Verification items for the finished model (mm, model axes). A direction names the side the tool comes from. Coordinates: 2 decimals unless noted, no trailing zeros. Loops run counter-clockwise (first coordinate to the right, second up) from the corner with the lowest first, then second, coordinate; pieces in that order, holes last.
Q1. Go/stop test with flat-tipped pins: P1, Ø3, axis at x = 57, y = 18.5, coming from the +Z side; P2, Ø5, axis at x = 78, z = -46.5, coming from the +Y side; P3, Ø4, axis at y = 19, z = -25, coming from the +X side; P4, Ø3, axis at y = 20.5, z = -59, coming from the +X side. Record where each tip stops, or that it passes through.
Q2. Sectioned sample at B-B (x = 66.5). Enter the section's corners in (y, z), then the cut area to 3 significant figures.
Q3. Sectioned sample at C-C (z = -9). Enter the section's corners in (x, y).
Q4. Sectioned sample at D-D (x = 9). Enter the section's corners in (y, z), then the cut area to 3 significant figures.
Q5. Material ranges on probe 1 along Y at (x, z) = (82, -53); probe 2 along Z at (x, y) = (54, 13.25); probe 3 along Z at (x, y) = (34, 3.5), recorded low to high.
Q6. Mould release check, pull along Z, two halves, no side actions. Record for faces 4 (the face through (60.53, 2.61, -50.89)), 5 (the face through (62.13, 2.85, -43.01)), 6 (the face through (23.49, 2.85, -19.79)): +Z half, -Z half, draft (parallel to the pull), parting line (faces both ways), or undercut.
Q7. Access from +Z, -Z, +X, -X, +Y, -Y to the whole of each face (thin tool, end or side, straight path). Record for faces 1 (the face through (26.5, 13, -20)), 2 (the face through (2.36, 13.73, -20.34)), 3 (the face through (62.13, 23.49, -42.85)).
Q8. Sectioned sample at A-A (y = 13.25). Enter the section's corners in (x, z), then the cut area to 3 significant figures.
```python
from build123d import *

# Parameters (mm, degrees)
BOSS_EXTRUDE1_DEPTH = 26.5
SKETCH3_R           = 10.9
CUT_EXTRUDE1_DEPTH  = 129.322835068
SKETCH4_R           = 10.9
CUT_EXTRUDE2_DEPTH  = 129.322835068
FILLET1_R           = 10


with BuildPart() as part:
    # Sketch2 → Boss-Extrude1 (new body)
    with BuildSketch(Plane(origin=(0, 0, 0), x_dir=(1, 0, 0), z_dir=(0, 1, 0))):
        Polygon((0, 0), (0, 66.5), (106.5, 66.5), (106.5, 40), (26.5, 40), (26.5, 0), align=None)
    extrude(amount=BOSS_EXTRUDE1_DEPTH)

    # Sketch3 → Cut-Extrude1 (cut, through all)
    with BuildSketch(Plane.XY):
        with Locations((13.25, 13.25)):
            Circle(SKETCH3_R)
    extrude(amount=-CUT_EXTRUDE1_DEPTH, mode=Mode.SUBTRACT)

    # Sketch4 → Cut-Extrude2 (cut, through all)
    with BuildSketch(Plane(origin=(106.5, 0, 0), x_dir=(0, 0, -1), z_dir=(1, 0, 0))):
        with Locations((53.25, 13.25)):
            Circle(SKETCH4_R)
    extrude(amount=-CUT_EXTRUDE2_DEPTH, mode=Mode.SUBTRACT)

    # Fillet1
    # the kernel refuses this fillet: 10 mm, written as the material it takes off along each edge
    with BuildSketch(Plane(origin=(106.5, 26.5, -40), x_dir=(0, 0, -1), z_dir=(-1, 0, 0))) as fillet1_piece_1:
        with BuildLine():
            CenterArc((FILLET1_R, FILLET1_R), FILLET1_R, 180, 90)
            Line((0, FILLET1_R), (-FILLET1_R * 0.02, FILLET1_R))
            Line((-FILLET1_R * 0.02, FILLET1_R), (-FILLET1_R * 0.02, -FILLET1_R * 0.02))
            Line((-FILLET1_R * 0.02, -FILLET1_R * 0.02), (FILLET1_R, -FILLET1_R * 0.02))
            Line((FILLET1_R, -FILLET1_R * 0.02), (FILLET1_R, 0))
        make_face()
    extrude(amount=80, mode=Mode.SUBTRACT)
    with BuildSketch(Plane(origin=(0, 26.5, -66.5), x_dir=(0, 0, 1), z_dir=(1, 0, 0))) as fillet1_piece_2:
        with BuildLine():
            CenterArc((FILLET1_R, FILLET1_R), FILLET1_R, 180, 90)
            Line((0, FILLET1_R), (-FILLET1_R * 0.02, FILLET1_R))
            Line((-FILLET1_R * 0.02, FILLET1_R), (-FILLET1_R * 0.02, -FILLET1_R * 0.02))
            Line((-FILLET1_R * 0.02, -FILLET1_R * 0.02), (FILLET1_R, -FILLET1_R * 0.02))
            Line((FILLET1_R, -FILLET1_R * 0.02), (FILLET1_R, 0))
        make_face()
    extrude(amount=106.5, mode=Mode.SUBTRACT)
    with BuildSketch(Plane(origin=(0, 0, -66.5), x_dir=(0, 0, 1), z_dir=(1, 0, 0))) as fillet1_piece_3:
        with BuildLine():
            CenterArc((FILLET1_R, -FILLET1_R), FILLET1_R, 90, 90)
            Line((0, -FILLET1_R), (-FILLET1_R * 0.02, -FILLET1_R))
            Line((-FILLET1_R * 0.02, -FILLET1_R), (-FILLET1_R * 0.02, FILLET1_R * 0.02))
            Line((-FILLET1_R * 0.02, FILLET1_R * 0.02), (FILLET1_R, FILLET1_R * 0.02))
            Line((FILLET1_R, FILLET1_R * 0.02), (FILLET1_R, 0))
        make_face()
    extrude(amount=106.5, mode=Mode.SUBTRACT)
    with BuildSketch(Plane(origin=(106.5, 0, -40), x_dir=(0, 0, -1), z_dir=(-1, 0, 0))) as fillet1_piece_4:
        with BuildLine():
            CenterArc((FILLET1_R, -FILLET1_R), FILLET1_R, 90, 90)
            Line((0, -FILLET1_R), (-FILLET1_R * 0.02, -FILLET1_R))
            Line((-FILLET1_R * 0.02, -FILLET1_R), (-FILLET1_R * 0.02, FILLET1_R * 0.02))
            Line((-FILLET1_R * 0.02, FILLET1_R * 0.02), (FILLET1_R, FILLET1_R * 0.02))
            Line((FILLET1_R, FILLET1_R * 0.02), (FILLET1_R, 0))
        make_face()
    extrude(amount=80, mode=Mode.SUBTRACT)
    with BuildSketch(Plane(origin=(26.5, 0, -40), x_dir=(-1, 0, 0), z_dir=(0, 0, 1))) as fillet1_piece_5:
        with BuildLine():
            CenterArc((FILLET1_R, -FILLET1_R), FILLET1_R, 90, 90)
            Line((0, -FILLET1_R), (-FILLET1_R * 0.02, -FILLET1_R))
            Line((-FILLET1_R * 0.02, -FILLET1_R), (-FILLET1_R * 0.02, FILLET1_R * 0.02))
            Line((-FILLET1_R * 0.02, FILLET1_R * 0.02), (FILLET1_R, FILLET1_R * 0.02))
            Line((FILLET1_R, FILLET1_R * 0.02), (FILLET1_R, 0))
        make_face()
    extrude(amount=40, mode=Mode.SUBTRACT)
    with BuildSketch(Plane(origin=(26.5, 26.5, -40), x_dir=(-1, 0, 0), z_dir=(0, 0, 1))) as fillet1_piece_6:
        with BuildLine():
            CenterArc((FILLET1_R, FILLET1_R), FILLET1_R, 180, 90)
            Line((0, FILLET1_R), (-FILLET1_R * 0.02, FILLET1_R))
            Line((-FILLET1_R * 0.02, FILLET1_R), (-FILLET1_R * 0.02, -FILLET1_R * 0.02))
            Line((-FILLET1_R * 0.02, -FILLET1_R * 0.02), (FILLET1_R, -FILLET1_R * 0.02))
            Line((FILLET1_R, -FILLET1_R * 0.02), (FILLET1_R, 0))
        make_face()
    extrude(amount=40, mode=Mode.SUBTRACT)
    with BuildSketch(Plane(origin=(106.5, 26.5, -40), x_dir=(0, 0, -1), z_dir=(-1, 0, 0))) as fillet1_piece_7a_section:
        with BuildLine():
            CenterArc((FILLET1_R, FILLET1_R), FILLET1_R, 180, 90)
            Line((0, FILLET1_R), (-FILLET1_R * 0.02, FILLET1_R))
            Line((-FILLET1_R * 0.02, FILLET1_R), (-FILLET1_R * 0.02, -FILLET1_R * 0.02))
            Line((-FILLET1_R * 0.02, -FILLET1_R * 0.02), (FILLET1_R, -FILLET1_R * 0.02))
            Line((FILLET1_R, -FILLET1_R * 0.02), (FILLET1_R, 0))
        make_face()
    fillet1_piece_7a = extrude(amount=105, mode=Mode.PRIVATE)
    fillet1_piece_7a = split(fillet1_piece_7a, bisect_by=Plane(origin=(26.5, 24.236048857, -42.263951143), z_dir=(-1, 0, 0)), keep=Keep.TOP, mode=Mode.PRIVATE)
    with BuildSketch(Plane(origin=(26.5, 26.5, -65), x_dir=(-1, 0, 0), z_dir=(0, 0, 1))) as fillet1_piece_7b_section:
        with BuildLine():
            CenterArc((FILLET1_R, FILLET1_R), FILLET1_R, 180, 90)
            Line((0, FILLET1_R), (-FILLET1_R * 0.02, FILLET1_R))
            Line((-FILLET1_R * 0.02, FILLET1_R), (-FILLET1_R * 0.02, -FILLET1_R * 0.02))
            Line((-FILLET1_R * 0.02, -FILLET1_R * 0.02), (FILLET1_R, -FILLET1_R * 0.02))
            Line((FILLET1_R, -FILLET1_R * 0.02), (FILLET1_R, 0))
        make_face()
    fillet1_piece_7b = extrude(amount=65, mode=Mode.PRIVATE)
    fillet1_piece_7b = split(fillet1_piece_7b, bisect_by=Plane(origin=(24.236048857, 24.236048857, -40), z_dir=(0, 0, -1)), keep=Keep.TOP, mode=Mode.PRIVATE)
    fillet1_piece_7 = fillet1_piece_7a & fillet1_piece_7b
    add(fillet1_piece_7, mode=Mode.SUBTRACT)
    with BuildSketch(Plane(origin=(106.5, 0, -40), x_dir=(0, 0, -1), z_dir=(-1, 0, 0))) as fillet1_piece_8a_section:
        with BuildLine():
            CenterArc((FILLET1_R, -FILLET1_R), FILLET1_R, 90, 90)
            Line((0, -FILLET1_R), (-FILLET1_R * 0.02, -FILLET1_R))
            Line((-FILLET1_R * 0.02, -FILLET1_R), (-FILLET1_R * 0.02, FILLET1_R * 0.02))
            Line((-FILLET1_R * 0.02, FILLET1_R * 0.02), (FILLET1_R, FILLET1_R * 0.02))
            Line((FILLET1_R, FILLET1_R * 0.02), (FILLET1_R, 0))
        make_face()
    fillet1_piece_8a = extrude(amount=105, mode=Mode.PRIVATE)
    fillet1_piece_8a = split(fillet1_piece_8a, bisect_by=Plane(origin=(26.5, 2.263951143, -42.263951143), z_dir=(-1, 0, 0)), keep=Keep.TOP, mode=Mode.PRIVATE)
    with BuildSketch(Plane(origin=(26.5, 0, -65), x_dir=(-1, 0, 0), z_dir=(0, 0, 1))) as fillet1_piece_8b_section:
        with BuildLine():
            CenterArc((FILLET1_R, -FILLET1_R), FILLET1_R, 90, 90)
            Line((0, -FILLET1_R), (-FILLET1_R * 0.02, -FILLET1_R))
            Line((-FILLET1_R * 0.02, -FILLET1_R), (-FILLET1_R * 0.02, FILLET1_R * 0.02))
            Line((-FILLET1_R * 0.02, FILLET1_R * 0.02), (FILLET1_R, FILLET1_R * 0.02))
            Line((FILLET1_R, FILLET1_R * 0.02), (FILLET1_R, 0))
        make_face()
    fillet1_piece_8b = extrude(amount=65, mode=Mode.PRIVATE)
    fillet1_piece_8b = split(fillet1_piece_8b, bisect_by=Plane(origin=(24.236048857, 2.263951143, -40), z_dir=(0, 0, -1)), keep=Keep.TOP, mode=Mode.PRIVATE)
    fillet1_piece_8 = fillet1_piece_8a & fillet1_piece_8b
    add(fillet1_piece_8, mode=Mode.SUBTRACT)


solid = part.part
```
Geometry check:
1. P1: stops at z = -40.01
1. P2: stops at y = 26.45
1. P3: stops at x = 26.49
1. P4: passes through
2. outline: (0, -56.5) arc R10 ccw to (10, -66.5) - (16.5, -66.5) arc R10 ccw to (26.5, -56.5) - (26.5, -50) arc R10 ccw to (16.5, -40) - (10, -40) arc R10 ccw to (0, -50) - close; hole circle Ø21.8 at (13.25, -53.25)
2. area: 243 mm2
3. outline: (0, 0) - (16.5, 0) arc R10 ccw to (26.5, 10) - (26.5, 16.5) arc R10 ccw to (16.5, 26.5) - (0, 26.5) - close; hole circle Ø21.8 at (13.25, 13.25)
4. outline: (0, -56.5) arc R10 ccw to (3.21, -63.84) - (3.21, -57.5) arc R10.9 cw to (3.21, -49) - (3.21, 0) - (0, 0) - close; (23.29, -63.84) arc R10 ccw to (26.5, -56.5) - (26.5, 0) - (23.29, 0) - (23.29, -49) arc R10.9 cw to (23.29, -57.5) - close
4. area: 386 mm2
5. probe 1: y = 0 to 2.35, 24.15 to 26.5
5. probe 2: z = -66.5 to -64.15, -42.35 to -40
5. probe 3: z = -64.1 to -58.12, -48.38 to -42.4
6. face 4: undercut
6. face 5: +Z half
6. face 6: draft
7. face 1: +Z, +X, +Y, -Y
7. face 2: +Z, -Z
7. face 3: +Z, +X, +Y
8. outline: (0, -66.5) - (2.35, -66.5) - (2.35, -64.15) - (0, -64.15) - close; (0, -42.35) - (2.35, -42.35) - (2.35, 0) - (0, 0) - close; (24.15, -66.5) - (106.5, -66.5) - (106.5, -64.15) - (24.15, -64.15) - close; (24.15, -42.35) - (106.5, -42.35) - (106.5, -40) - (26.5, -40) - (26.5, 0) - (24.15, 0) - close
8. area: 586 mm2
